Autodesk Inventor part; units mm, degrees
ref_plane "YZ Plane" through (0, 0, 0) normal (1, 0, 0) x (0, 1, 0)
ref_plane "XZ Plane" through (0, 0, 0) normal (0, 1, 0) x (-1, 0, 0)
ref_plane "XY Plane" through (0, 0, 0) normal (0, 0, 1) x (1, 0, 0)
sketch "Sketch1" plane through (0, 0, 0) normal (0, 0, 1) x (1, 0, 0)
  line L0 (107.9, 41.925) -> (107.9, -41.925)
  line L1 (-107.9, -41.925) -> (-107.9, 41.925)
  line L2 (-107.9, 41.925) -> (107.9, -41.925) construction
  line L3 (107.9, 41.925) -> (-107.9, -41.925) construction
  line L4 (-15.6, 80.925) -> (15.6, 80.925)
  line L5 (-15.6, 41.925) -> (-107.9, 41.925)
  line L6 (15.6, 41.925) -> (107.9, 41.925)
  line L7 (-107.9, -41.925) -> (-49.4, -67.398)
  line L8 (107.9, -41.925) -> (49.4, -67.398)
  line L9 (49.4, -67.398) -> (-49.4, -67.398)
  line L10 (-114.4, -47.125) -> (-114.4, 47.125)
  line L11 (114.4, 47.125) -> (114.4, -47.125)
  line L12 (114.4, -47.125) -> (-114.4, 47.125) construction
  line L13 (-114.4, -47.125) -> (114.4, 47.125) construction
  line L14 (-22.1, 47.125) -> (-22.1, 86.125)
  line L15 (-22.1, 86.125) -> (22.1, 86.125)
  line L16 (22.1, 86.125) -> (22.1, 47.125)
  line L17 (22.1, 47.125) -> (114.4, 47.125)
  line L18 (-22.1, 47.125) -> (-114.4, 47.125)
  line L19 (114.4, -47.125) -> (49.4, -75.4283)
  line L20 (-114.4, -47.125) -> (-49.4, -75.4283)
  line L21 (49.4, -75.4283) -> (-49.4, -75.4283)
  line L22 (-15.6, 41.925) -> (-15.6, 80.925)
  line L23 (15.6, 41.925) -> (15.6, 80.925)
  point P0 (0, 0)
  point P1 (0, 0)
  point P2 (0, 80.925)
  point P3 (0, 0)
  point P4 (0, 86.125)
  point P5 (0, 0)
  dimension "Comp" = 215.8
  dimension "Lar" = 83.85
  dimension "Larg1" = 31.2
  dimension "d10" = 215.8
  dimension "d15" = 58.5
  dimension "d16" = 98.8
  dimension "d17" = 58.5
  dimension "LarMaior" = 94.25
  dimension "CompMaior" = 228.8
  dimension "d20" = 39
  dimension "d21" = 44.2
  dimension "d22" = 39
  dimension "d25" = 65
  dimension "d27" = 65
  dimension "d28" = 98.8
extrude "Extrusion1" add sketch "Sketch1" along normal blind 6.5 contours L0 L8 L9 L7 L1 L5 L22 L4 L23 L6 | L10 L18 L14 L15 L16 L17 L11 L19 L21 L20
shell "Shell1" thickness 6.5 both sides yes removed faces 2 at (-7.3667, -34.5772, 6.5) at (-7.3667, -34.5772, 0)
properties part number "Buste1"
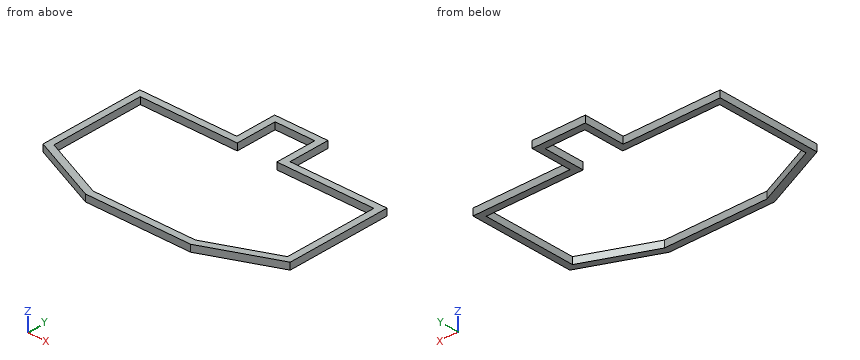
Verification items for the finished model (mm, model axes). Coordinates: 2 decimals unless noted, no trailing zeros. Loops run counter-clockwise (first coordinate to the right, second up) from the corner with the lowest first, then second, coordinate; pieces in that order, holes last. Notation, with made-up numbers: (22, 63.5) -> (46, 63.5) arc R11 ccw to (46, 72.5) -> close; hole circle Ø1 at (80, -32.75). An arc over 180 degrees is marked (long way). Answer as a JSON object with one key per item and string values. Group by question number.
Item 1: Sectioned sample at C-C on z = 3.5. Record the boundary of the cut face in (x, y) (3 decimals), plus the area to 3 significant figures.
Item 2: Scan lines: probe 1 along X at (y, z) = (6.5, 3.25); probe 2 along Y at (x, z) = (26, 1) (3 decimals); probe 3 along X at (y, z) = (62, 3). Record each from-to range of solid material in increasing order.
Item 3: Sectioned sample at A-A on y = 73.5. Record the boundary of the cut face in (x, z).
Item 4: Depth check by flat-ended pin: pin 1 (2 mm diameter, centred on y = 60.5, z = 4.5, fed in from +X); pin 2 (3 mm diameter, centred on x = -56.5, z = 2, fed in from +Y) (3 decimals); pin 3 (2 mm diameter, centred on y = 59.5, z = 3.5, fed in from -X). Enter the tip coordinate at first touch or a pass-through.
Item 5: Sectioned sample at B-B on x = 7. Record the boundary of the cut face in (y, z) (3 decimals).
Evaluation:
{
 "1": {"outline": "(-117.65, -49.255) -> (-50.077, -78.678) -> (50.077, -78.678) -> (117.65, -49.255) -> (117.65, 50.375) -> (25.35, 50.375) -> (25.35, 89.375) -> (-25.35, 89.375) -> (-25.35, 50.375) -> (-117.65, 50.375) -> close; hole (-111.15, -44.995) -> (-48.723, -72.178) -> (48.723, -72.178) -> (111.15, -44.995) -> (111.15, 43.875) -> (18.85, 43.875) -> (18.85, 82.875) -> (-18.85, 82.875) -> (-18.85, 43.875) -> (-111.15, 43.875) -> close", "area": "4,780 mm²"},
 "2": {"probe 1": "x = -117.65 to -111.15, 111.15 to 117.65", "probe 2": "y = -78.678 to -72.178, 43.875 to 50.375", "probe 3": "x = -25.35 to -18.85, 18.85 to 25.35"},
 "3": {"outline": "(-25.35, 0) -> (-18.85, 0) -> (-18.85, 6.5) -> (-25.35, 6.5) -> close; (18.85, 0) -> (25.35, 0) -> (25.35, 6.5) -> (18.85, 6.5) -> close"},
 "4": {"pin 1": "stops at x = 25.35", "pin 2": "stops at y = 50.375", "pin 3": "stops at x = -25.35"},
 "5": {"outline": "(-78.678, 0) -> (-72.178, 0) -> (-72.178, 6.5) -> (-78.678, 6.5) -> close; (82.875, 0) -> (89.375, 0) -> (89.375, 6.5) -> (82.875, 6.5) -> close"}
}
